```python
from build123d import *

# Parameters (mm, degrees)
CYLINDER012_R     = 2
CYLINDER012_DEPTH = 5
CYLINDER011_R     = 2.75
CYLINDER011_DEPTH = 4
CYLINDER010_R     = 2
CYLINDER010_DEPTH = 5
CYLINDER009_R     = 2.75
CYLINDER009_DEPTH = 4
CYLINDER008_R     = 2
CYLINDER008_DEPTH = 5
CYLINDER007_R     = 2.75
CYLINDER007_DEPTH = 4
CYLINDER014_R     = 2
CYLINDER014_DEPTH = 5
CYLINDER013_R     = 2.75
CYLINDER013_DEPTH = 4
CYLINDER006_R     = 11
CYLINDER006_DEPTH = 5
BOX005_W          = 42.3
BOX005_H          = 42.3
BOX005_DEPTH      = 5


with BuildPart() as cylinder012:
    # Cylinder012 → Cylinder012 (new body)
    with BuildSketch(Plane.XY.offset(-5)):
        Circle(CYLINDER012_R)
    extrude(amount=CYLINDER012_DEPTH)


with BuildPart() as fusion004:
    # Cylinder011 → Cylinder011 (new body)
    with BuildSketch(Plane.XY.offset(-5)):
        Circle(CYLINDER011_R)
    extrude(amount=CYLINDER011_DEPTH)

    # Fusion004: union Cylinder012
    add(cylinder012.part)


with BuildPart() as fusion004_1:
    # Fusion004 placement: moved
    add(fusion004.part.moved(Location((-15.5, 15.5, 0))))


with BuildPart() as cylinder010:
    # Cylinder010 → Cylinder010 (new body)
    with BuildSketch(Plane.XY.offset(-5)):
        Circle(CYLINDER010_R)
    extrude(amount=CYLINDER010_DEPTH)


with BuildPart() as fusion003:
    # Cylinder009 → Cylinder009 (new body)
    with BuildSketch(Plane.XY.offset(-5)):
        Circle(CYLINDER009_R)
    extrude(amount=CYLINDER009_DEPTH)

    # Fusion003: union Cylinder010
    add(cylinder010.part)


with BuildPart() as fusion003_1:
    # Fusion003 placement: moved
    add(fusion003.part.moved(Location((15.5, -15.5, 0))))


with BuildPart() as cylinder008:
    # Cylinder008 → Cylinder008 (new body)
    with BuildSketch(Plane.XY.offset(-5)):
        Circle(CYLINDER008_R)
    extrude(amount=CYLINDER008_DEPTH)


with BuildPart() as fusion002:
    # Cylinder007 → Cylinder007 (new body)
    with BuildSketch(Plane.XY.offset(-5)):
        Circle(CYLINDER007_R)
    extrude(amount=CYLINDER007_DEPTH)

    # Fusion002: union Cylinder008
    add(cylinder008.part)


with BuildPart() as fusion002_1:
    # Fusion002 placement: moved
    add(fusion002.part.moved(Location((-15.5, -15.5, 0))))


with BuildPart() as cylinder014:
    # Cylinder014 → Cylinder014 (new body)
    with BuildSketch(Plane.XY.offset(-5)):
        Circle(CYLINDER014_R)
    extrude(amount=CYLINDER014_DEPTH)


with BuildPart() as compound006:
    # Cylinder013 → Cylinder013 (new body)
    with BuildSketch(Plane.XY.offset(-5)):
        Circle(CYLINDER013_R)
    extrude(amount=CYLINDER013_DEPTH)

    # Fusion005: union Cylinder014
    add(cylinder014.part)


with BuildPart() as compound006_1:
    # Fusion005 placement: moved
    add(compound006.part.moved(Location((15.5, 15.5, 0))))

    # Compound006: union Fusion004, Fusion003, Fusion002
    add(fusion004_1.part)
    add(fusion003_1.part)
    add(fusion002_1.part)


with BuildPart() as cylinder006:
    # Cylinder006 → Cylinder006 (new body)
    with BuildSketch(Plane.XY.offset(-5)):
        Circle(CYLINDER006_R)
    extrude(amount=CYLINDER006_DEPTH)


with BuildPart() as cut003:
    # Box005 → Box005 (new body)
    with BuildSketch(Plane(origin=(-21.15, -21.15, -5), x_dir=(1, 0, 0), z_dir=(0, 0, 1))):
        with Locations((21.15, 21.15)):
            Rectangle(BOX005_W, BOX005_H)
    extrude(amount=BOX005_DEPTH)

    # Cut002: cut Cylinder006
    add(cylinder006.part, mode=Mode.SUBTRACT)

    # Cut003: cut Compound006
    add(compound006_1.part, mode=Mode.SUBTRACT)


solid = cut003.part
```
Check sheet for the modelled part. Datum: model origin and axes. Units: mm. A direction names the side the tool comes from. Coordinates: 2 decimals unless noted, no trailing zeros. Write each loop counter-clockwise with the first axis right and the second up, starting at its lowest first coordinate (ties: lowest second). Pieces come first, ordered by that corner, then holes. Notation, with made-up numbers: (47, 10.25) - (91, 10.25) arc R12 cw to (91, 15.25) - close; hole circle Ø8 at (-35, 8). An arc over 180 degrees is marked (long way). One line per question, with ' | ' between items.
Item 1: Sectioned sample at B-B on y = 0. Record the boundary of the cut face in (x, z), plus the area to 4 significant figures.
Determined:
outline: (-21.15, -5) - (-11, -5) - (-11, 0) - (-21.15, 0) - close; (11, -5) - (21.15, -5) - (21.15, 0) - (11, 0) - close | area: 101.5 mm2
Item 2: Mould release check, pull along X, two halves, no side actions. Record for faces 3 (the face through (16, 13, -1)), 4 (the face through (-21.15, 0, -3)), 5 (the face through (-10, -9, -5)): pulls with the +X half, pulls with the -X half, needs draft (parallel to the pull), parting line crosses it, or undercut.
Determined:
face 3: undercut | face 4: pulls with the -X half | face 5: needs draft
Item 3: Sectioned sample at C-C on z = -3.05. Record the boundary of the cut face in (x, y), plus the area to 3 significant figures.
Determined:
outline: (-21.15, -21.15) - (21.15, -21.15) - (21.15, 21.15) - (-21.15, 21.15) - close; hole circle Ø5.5 at (-15.5, -15.5); hole circle Ø5.5 at (-15.5, 15.5); hole circle Ø22 at (0, 0); hole circle Ø5.5 at (15.5, -15.5); hole circle Ø5.5 at (15.5, 15.5) | area: 1,310 mm2
Item 4: Gauge pin test, flat end, axial feed: P1, Ø5, axis at x = -15.5, y = -15.5, coming from the -Z side. Record the tip position at first contact, or that the pin passes through.
Determined:
P1: stops at z = -1
Item 5: Sectioned sample at A-A on x = 15.5. Record the boundary of the cut face in (y, z).
Determined:
outline: (-21.15, -5) - (-18.25, -5) - (-18.25, -1) - (-17.5, -1) - (-17.5, 0) - (-21.15, 0) - close; (-13.5, -1) - (-12.75, -1) - (-12.75, -5) - (12.75, -5) - (12.75, -1) - (13.5, -1) - (13.5, 0) - (-13.5, 0) - close; (17.5, -1) - (18.25, -1) - (18.25, -5) - (21.15, -5) - (21.15, 0) - (17.5, 0) - close
Item 6: Access from +Z, -Z, +X, -X, +Y, -Y to the whole of each face (thin tool, end or side, straight path). Record for faces 1 (the face through (15.24, -13.517, -0.507)), 2 (the face through (16, -18, -1)).
Determined:
face 1: +Z, -Z | face 2: -Z
Item 7: Thickness scan on line 1 (X direction, y = -15.5, z = -0.5); line 2 (X direction, y = 15, z = -4.1). Record the ranges inside material, lowest first. Write a range as [from, to].
Determined:
line 1: x = [-21.15, -17.5], [-13.5, 13.5], [17.5, 21.15] | line 2: x = [-21.15, -18.2], [-12.8, 12.8], [18.2, 21.15]
